Part model, mm, in its own coordinate system. Face numbers are marked on the shaded views. Give positions to 0.01 mm unless a question says otherwise; leave off trailing zeros. Loops run counter-clockwise (first coordinate to the right, second up) from the corner with the lowest first, then second, coordinate; pieces in that order, holes last. Notation, with made-up numbers: (76, 11) -> (132, 11) arc R14 ccw to (132, 37) -> close; hole circle Ø5 at (75.5, 57). An arc over 180 degrees is marked (long way). One line per question, with ' | ' between items.
```python
from build123d import *

# Parameters (mm, degrees)
F0_R     = 12.7
F1_DEPTH = 12.7
F3_D     = 6.35
F3_DEPTH = 12.7
F3_TIP   = 1.9077324654


with BuildPart() as f1:
    # F0 (on Front) → F1 (new body, symmetric)
    with BuildSketch(Plane.XZ):
        with BuildLine():
            Line((19.05, -25.4), (19.05, 0))
            ThreePointArc((19.05, 0), (0, 19.05), (-19.05, 0))
            Line((-19.05, 0), (-19.05, -25.4))
            Line((-19.05, -25.4), (19.05, -25.4))
        make_face()
        Circle(F0_R, mode=Mode.SUBTRACT)
    extrude(amount=F1_DEPTH, both=True)

    # F3
    with Locations(Plane(origin=(0, 0, -25.4), x_dir=(1, 0, 0), z_dir=(0, 0, -1))):
        with Locations((-12.7, 0), (12.7, 0)):
            Hole(F3_D / 2, depth=F3_DEPTH)
            with Locations((0, 0, -(F3_DEPTH + F3_TIP / 2))):  # 118° drill point
                Cone(0, F3_D / 2, F3_TIP, mode=Mode.SUBTRACT)


solid = f1.part
```
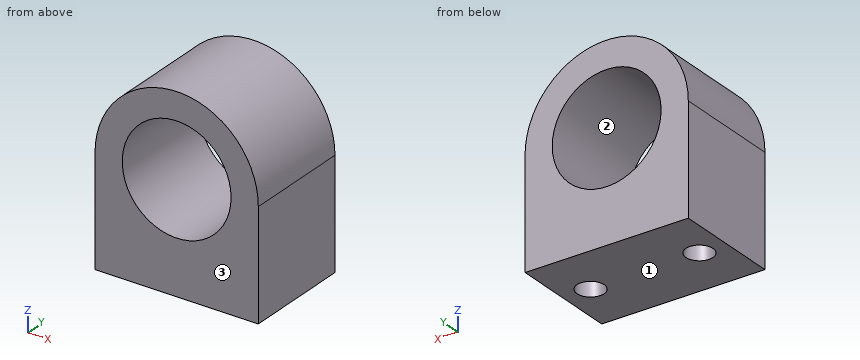
1) Saw through at B-B (x = 0). Give the cut face in (y, z).
Found:
outline: (-12.7, -25.4) -> (12.7, -25.4) -> (12.7, -12.7) -> (-12.7, -12.7) -> close; (-12.7, 12.7) -> (12.7, 12.7) -> (12.7, 19.05) -> (-12.7, 19.05) -> close
2) Pull direction Z, two halves, no side cores. Call the marked faces 1, 2 and 3: pulls with the +Z half, pulls with the -Z half, needs draft (parallel to the pull), parting line crosses it, or undercut.
Found:
face 1: pulls with the -Z half | face 2: undercut | face 3: needs draft
3) Saw through at C-C (y = 5). Give the cut face in (x, z).
Found:
outline: (-19.05, -25.4) -> (19.05, -25.4) -> (19.05, 0) arc R19.05 ccw to (-19.05, 0) -> close; hole circle Ø25.4 at (0, 0)
4) Drill centre lines: line 1 (Z direction, x = 0, y = 5); line 2 (Y direction, x = 12.7, z = -22.5) (3 decimals); line 3 (Y direction, x = -12, z = -18). Where is each one in solid material? Low to high.
Found:
line 1: -25.4 to -12.7, 12.7 to 19.05 | line 2: -12.7 to -3.175, 3.175 to 12.7 | line 3: -12.7 to -3.1, 3.1 to 12.7
5) Saw through at D-D (z = -3). Give the cut face in (x, y).
Found:
outline: (-19.05, -12.7) -> (-12.34, -12.7) -> (-12.34, 12.7) -> (-19.05, 12.7) -> close; (12.34, -12.7) -> (19.05, -12.7) -> (19.05, 12.7) -> (12.34, 12.7) -> close
6) Pin check, flat tips, straight feed: P1, Ø10, axis at x = -12.7, y = 0, coming from the +Z side; P2, Ø8, axis at x = 4, y = 8.5, coming from the +Z side; P3, Ø8.5, axis at x = 12.7, y = 0, coming from the +Z side. Stop position of each tip, or through.
Found:
P1: z = 17.42 | P2: z = 19.05 | P3: z = 17.07
7) Saw through at A-A (z = -11.5). Give the cut face in (x, y).
Found:
outline: (-19.05, -12.7) -> (-5.39, -12.7) -> (-5.39, 12.7) -> (-19.05, 12.7) -> close; (5.39, -12.7) -> (19.05, -12.7) -> (19.05, 12.7) -> (5.39, 12.7) -> close; hole circle Ø2.36 at (-12.7, 0); hole circle Ø2.36 at (12.7, 0)
